from build123d import *

# Parameters (mm, degrees)
CHAMFER1_SIZE            = 1
CHAMFER2_SIZE            = 1
SKETCH3_R                = 4
CUT_EXTRUDE1_DEPTH       = 178.676672639
CUT_EXTRUDE2_START       = -3
CUT_EXTRUDE2_DEPTH       = 14
BOSS_EXTRUDE1_REACH      = 181.148
BOSS_EXTRUDE1_END_RADIUS = 9


with BuildPart() as part:
    # Sketch2 → Revolve1 (revolve)
    with BuildSketch(Plane(origin=(0, 0, 0), x_dir=(0, 0, -1), z_dir=(1, 0, 0))):
        Polygon((0, 0), (50, 0), (50, 13), (25, 13), (25, 23), (10, 23), (10, 143), (9, 143), (9, 163), (0, 163), align=None)
    revolve(axis=Axis((0, 0, 0), (0, 1, 0)))

    # Chamfer1
    chamfer1_edges = [part.edges().sort_by_distance(p)[0] for p in [
        (0, 163, 9),
    ]]
    chamfer(chamfer1_edges, length=CHAMFER1_SIZE)

    # Chamfer2
    chamfer2_edges = [part.edges().sort_by_distance(p)[0] for p in [
        (0, 23, 25),
    ]]
    chamfer(chamfer2_edges, length=CHAMFER2_SIZE)

    # Sketch3 → Cut-Extrude1 (cut, through all)
    with BuildSketch(Plane.XZ):
        with Locations(Location((40, 0, 0), (0, 0, 270))):
            Circle(SKETCH3_R)
        with Locations(Location((28.284271247, -28.284271247, 0), (0, 0, 270))):
            Circle(SKETCH3_R)
        with Locations(Location((0, -40, 0), (0, 0, 270))):
            Circle(SKETCH3_R)
        with Locations(Location((-28.284271247, -28.284271247, 0), (0, 0, 270))):
            Circle(SKETCH3_R)
        with Locations(Location((-40, 0, 0), (0, 0, 270))):
            Circle(SKETCH3_R)
        with Locations(Location((-28.284271247, 28.284271247, 0), (0, 0, 270))):
            Circle(SKETCH3_R)
        with Locations(Location((0, 40, 0), (0, 0, 270))):
            Circle(SKETCH3_R)
        with Locations(Location((28.284271247, 28.284271247, 0), (0, 0, 270))):
            Circle(SKETCH3_R)
    extrude(amount=-CUT_EXTRUDE1_DEPTH, mode=Mode.SUBTRACT)

    # Sketch5 → Cut-Extrude2 (cut)
    with BuildSketch(Plane(origin=(0, 163, 0), x_dir=(1, 0, 0), z_dir=(0, 1, 0)).offset(CUT_EXTRUDE2_START)):
        with BuildLine():
            Line((-3, 5), (3, 5))
            Line((3, 5), (3, 8.485281374))
            ThreePointArc((3, 8.485281374), (0, 9), (-3, 8.485281374))
            Line((-3, 8.485281374), (-3, 5))
        make_face()
    extrude(amount=-CUT_EXTRUDE2_DEPTH, mode=Mode.SUBTRACT)

    # Boss-Extrude1: up to this cylinder (the profile starts inside it)
    boss_extrude1_end = Plane(origin=(0, 153, 0), z_dir=(0, -1, 0)) * Cylinder(BOSS_EXTRUDE1_END_RADIUS, 381.296, mode=Mode.PRIVATE)
    # Sketch6 → Boss-Extrude1 (add, up to the surface)
    with BuildSketch(Plane(origin=(0, 0, -5), x_dir=(-1, 0, 0), z_dir=(0, 0, -1)), mode=Mode.PRIVATE) as boss_extrude1_sk1:
        with BuildLine():
            ThreePointArc((-2, 158), (-1.414213562, 159.414213562), (0, 160))
            Line((0, 160), (-3, 160))
            Line((-3, 160), (-3, 146))
            Line((-3, 146), (0, 146))
            ThreePointArc((0, 146), (-1.414213562, 146.585786438), (-2, 148))
            Line((-2, 148), (-2, 158))
        make_face()
    boss_extrude1_tool1 = extrude(boss_extrude1_sk1.sketch, amount=BOSS_EXTRUDE1_REACH, mode=Mode.PRIVATE) & boss_extrude1_end
    add(boss_extrude1_tool1.solids().sort_by_distance((2.396584, 153, -5))[0])
    # Sketch6 → Boss-Extrude1 (add, up to the surface)
    with BuildSketch(Plane(origin=(0, 0, -5), x_dir=(-1, 0, 0), z_dir=(0, 0, -1)), mode=Mode.PRIVATE) as boss_extrude1_sk2:
        with BuildLine():
            Line((3, 160), (0, 160))
            ThreePointArc((0, 160), (1.414213562, 159.414213562), (2, 158))
            Line((2, 158), (2, 148))
            ThreePointArc((2, 148), (1.414213562, 146.585786438), (0, 146))
            Line((0, 146), (3, 146))
            Line((3, 146), (3, 160))
        make_face()
    boss_extrude1_tool2 = extrude(boss_extrude1_sk2.sketch, amount=BOSS_EXTRUDE1_REACH, mode=Mode.PRIVATE) & boss_extrude1_end
    add(boss_extrude1_tool2.solids().sort_by_distance((-2.396584, 153, -5))[0])


solid = part.part
Here's how the part is built. I have some questions about the finished solid (model axes, mm). A direction names the side the tool comes from. Round coordinates to 2 decimals unless told otherwise and drop trailing zeros. Loops run counter-clockwise (first coordinate to the right, second up) from the corner with the lowest first, then second, coordinate; pieces in that order, holes last. Notation, with made-up numbers: (72.5, 62.25) - (123.5, 62.25) arc R28 ccw to (123.5, 90.25) - close; hole circle Ø8 at (54.25, 89.5). An arc over 180 degrees is marked (long way). One line per question, with ' | ' between items. Start each with the question number.
Q1. We'd pull the mould along X, two halves only. Please class faces 4 (the cylindrical face through (9.76, 83.84, 2.17)), 5 (the flat face through (-2, 143, 9)), 6 (the flat face through (-2, 153, -7)): +X half, -X half, draft (parallel to the pull), parting line (faces both ways), or undercut.
Q2. Please list where these lines run through material, in increasing order: line 1 (X direction, y = 3, z = 0); line 2 (Y direction, x = -17, z = 26.5); line 3 (X direction, y = 9, z = -40). Write a range as [from, to].
Q3. I want a section at A-A (z = 0). Write out the boundary of the cut face in (x, y), then the cut area to 3 significant figures.
Q4. For faces 1 (the cylindrical face through (30.99, 6.41, 31.23)), 2 (the flat face through (-0.3, 23, -10.3)), 3 (the flat face through (0, 153, -5)), which set-ups out of +Z, -Z, +X, -X, +Y, -Y let a thin tool reach every point of the face, with its end or its side?
Q5. I want a section at C-C (z = -40). Write out the boundary of the cut face in (x, y).
Q6. Will these pins go through, and if not, where does the flat tip stop? pin 1 (13 mm diameter, centred on x = 28.28, z = 28.28, fed in from +Y); pin 2 (4 mm diameter, centred on y = 153.5, z = -7, fed in from +X); pin 3 (3 mm diameter, centred on x = 15, y = 17.5, fed in from +Z).
Q7. I want a section at B-B (x = -40). Write out the boundary of the cut face in (y, z), then the cut area to 3 significant figures.
Response values:
1) face 4: parting line | face 5: draft | face 6: undercut
2) line 1: x = [-50, -44], [-36, 36], [44, 50] | line 2: y = [0, 13] | line 3: x = [-30, -4], [4, 30]
3) outline: (-50, 0) - (-44, 0) - (-44, 13) - (-50, 13) - close; (-36, 0) - (36, 0) - (36, 13) - (25, 13) - (25, 22) - (24, 23) - (10, 23) - (10, 143) - (9, 143) - (9, 162) - (8, 163) - (-8, 163) - (-9, 162) - (-9, 143) - (-10, 143) - (-10, 23) - (-24, 23) - (-25, 22) - (-25, 13) - (-36, 13) - close; (44, 0) - (50, 0) - (50, 13) - (44, 13) - close | area: 4,350 mm²
4) face 1: +Y, -Y | face 2: +Y | face 3: -Z
5) outline: (-30, 0) - (-4, 0) - (-4, 13) - (-30, 13) - close; (4, 0) - (30, 0) - (30, 13) - (4, 13) - close
6) pin 1: stops at y = 13 | pin 2: stops at x = 7.48 | pin 3: stops at z = 21.04
7) outline: (0, -30) - (13, -30) - (13, -4) - (0, -4) - close; (0, 4) - (13, 4) - (13, 30) - (0, 30) - close | area: 676 mm²
